from build123d import *

# Parameters (mm, degrees)
SKETCH2_R           = 2.159
BOSS_EXTRUDE2_DEPTH = 2.286


with BuildPart() as part:
    # Sketch2 → Boss-Extrude2 (new body)
    with BuildSketch(Plane(origin=(0, 0, 0), x_dir=(1, 0, 0), z_dir=(0, 1, 0))):
        with BuildLine():
            Line((-39.486864346, -27.37374707), (-39.486864346, 37.14225293))
            Line((-39.486864346, 37.14225293), (-36.946864346, 39.68225293))
            Line((-36.946864346, 39.68225293), (27.569135654, 39.68225293))
            Line((27.569135654, 39.68225293), (30.109135654, 37.14225293))
            Line((30.109135654, 37.14225293), (30.109135654, 16.82225293))
            Line((30.109135654, 16.82225293), (27.569135654, 14.28225293))
            Line((27.569135654, 14.28225293), (-7.736864346, 14.28225293))
            ThreePointArc((-7.736864346, 14.28225293), (-12.226992406, 12.422380991), (-14.086864346, 7.93225293))
            Line((-14.086864346, 7.93225293), (-14.086864346, -27.37374707))
            Line((-14.086864346, -27.37374707), (-16.626864346, -29.91374707))
            Line((-16.626864346, -29.91374707), (-36.946864346, -29.91374707))
            Line((-36.946864346, -29.91374707), (-39.486864346, -27.37374707))
        make_face()
        with Locations((-26.786864346, 26.98225293)):
            Circle(SKETCH2_R, mode=Mode.SUBTRACT)
        with Locations((-14.086864346, 26.98225293)):
            Circle(SKETCH2_R, mode=Mode.SUBTRACT)
        with Locations((-1.386864346, 26.98225293)):
            Circle(SKETCH2_R, mode=Mode.SUBTRACT)
        with Locations((11.313135654, 26.98225293)):
            Circle(SKETCH2_R, mode=Mode.SUBTRACT)
        with Locations((24.013135654, 26.98225293)):
            Circle(SKETCH2_R, mode=Mode.SUBTRACT)
        with Locations((-26.786864346, 14.34575293)):
            Circle(SKETCH2_R, mode=Mode.SUBTRACT)
        with Locations((-26.786864346, 1.70925293)):
            Circle(SKETCH2_R, mode=Mode.SUBTRACT)
        with Locations((-26.786864346, -10.92724707)):
            Circle(SKETCH2_R, mode=Mode.SUBTRACT)
        with Locations((-26.786864346, -23.56374707)):
            Circle(SKETCH2_R, mode=Mode.SUBTRACT)
    extrude(amount=BOSS_EXTRUDE2_DEPTH)


solid = part.part
Here's how the part is built. I have some questions about the finished solid (model axes, mm). A direction names the side the tool comes from. Round coordinates to 2 decimals unless told otherwise and drop trailing zeros. Write each loop counter-clockwise with the first axis right and the second up, starting at its lowest first coordinate (ties: lowest second). Pieces come first, ordered by that corner, then holes.
1. Suppose I cut it at B-B (y = 0.8). State how many separate pieces and enclosed holes the cut face has, and give its area (3 significant figures).
2. If we mould it in two halves opening along Z, with no side actions, what happens to faces 1 (the cylindrical face through (-25.63, 1.13, 21.74)), 2 (the flat face through (-12, 2.286, -13)), 3 (the flat face through (28.857, 1.127, -15.57))? For each: released by +Z, released by -Z, zero draft, split by the parting line, or undercut.
3. Suppose I cut it at D-D (x = -5). List the corners of the cut face in (y, z) for me, and give its area (3 significant figures).
4. I need wall thicknesses on L1, parallel to X at y = 1.85, z = -27; L2, parallel to Z at x = 1, y = 1.5; L3, parallel to X at y = 0.55, z = 8. Which ranges of each line are inside material? Lowest first, please.
5. For faces 4 (the flat face through (10, 1, -14.282)), 5 (the flat face through (-12, 0, -13)), which set-ups out of +Z, -Z, +X, -X, +Y, -Y let a thin tool reach every point of the face, with its end or its side?
6. Suppose I cut it at C-C (z = 18). List the corners of the cut face in (x, y) for me, and give its area (3 significant figures).
7. Will these pins go through, and if not, where does the flat tip stop? pin 1 Ø3.5 at (x, z) = (-26.79, 23.56) entering from -Y; pin 2 Ø1.1 at (y, z) = (1, 17.5) entering from +X; pin 3 Ø1.1 at (x, y) = (12, 1.5) entering from +Z.
8. Suppose I cut it at A-A (x = -25.5). List the corners of the cut face in (y, z) for me, and give its area (3 significant figures).
Answer sheet:
1. separate pieces: 1
1. enclosed holes: 9
1. area: 2,750 mm2
2. face 1: undercut
2. face 2: zero draft
2. face 3: released by +Z
3. outline: (0, -39.68) - (2.29, -39.68) - (2.29, -14.28) - (0, -14.28) - close
3. area: 58.1 mm2
4. L1: x = -39.49 to -28.95, -24.63 to -16.25, -11.93 to -3.55, 0.77 to 9.15, 13.47 to 21.85, 26.17 to 30.11
4. L2: z = -39.68 to -14.28
4. L3: x = -39.49 to -14.09
5. face 4: +Z, +X, +Y, -Y
5. face 5: +Z, -Z, +X, -X, -Y
6. outline: (-39.49, 0) - (-14.09, 0) - (-14.09, 2.29) - (-39.49, 2.29) - close
6. area: 58.1 mm2
7. pin 1: passes through
7. pin 2: stops at x = -14.09
7. pin 3: stops at z = -14.28
8. outline: (0, -39.68) - (2.29, -39.68) - (2.29, -28.72) - (0, -28.72) - close; (0, -25.25) - (2.29, -25.25) - (2.29, -16.08) - (0, -16.08) - close; (0, -12.61) - (2.29, -12.61) - (2.29, -3.44) - (0, -3.44) - close; (0, 0.02) - (2.29, 0.02) - (2.29, 9.19) - (0, 9.19) - close; (0, 12.66) - (2.29, 12.66) - (2.29, 21.83) - (0, 21.83) - close; (0, 25.3) - (2.29, 25.3) - (2.29, 29.91) - (0, 29.91) - close
8. area: 119 mm2
